Work out the finished part from the listing and answer in its coordinate system (mm). Face numbers are marked on the shaded views. Coordinates: 2 decimals unless noted, no trailing zeros. Order: outer loops, then holes, each group sorted by start corner. A loop starts at its lowest first (then second) coordinate and runs counter-clockwise, first axis right, second up. Notation, with made-up numbers: M 79,39.25 L 120,39.25 A28 cw 120,76.25 Z; hole C 75.5,75 d8. An arc over 180 degrees is marked long. Use a Markdown table: item, result.
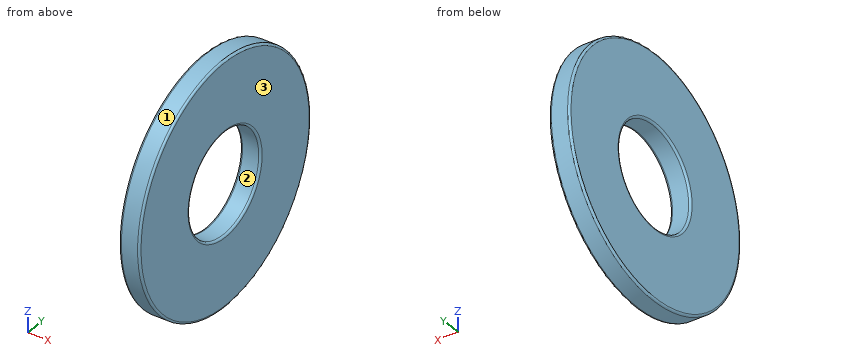
from build123d import *

# Parameters (mm, degrees)
F0_R     = 6
F0_R_2   = 2.5
F1_DEPTH = 1
F2_R     = 0.1
F3_R     = 0.1


with BuildPart() as f1:
    # F0 (on Right) → F1 (new body)
    with BuildSketch(Plane.YZ):
        Circle(F0_R)
        Circle(F0_R_2, mode=Mode.SUBTRACT)
    extrude(amount=F1_DEPTH)

    # F2
    f2_edges = [f1.edges().sort_by_distance(p)[0] for p in [
        (1, -6, 0),
        (0, -6, 0),
    ]]
    fillet(f2_edges, radius=F2_R)

    # F3
    f3_edges = [f1.edges().sort_by_distance(p)[0] for p in [
        (0, -2.5, 0),
        (1, -2.5, 0),
    ]]
    fillet(f3_edges, radius=F3_R)


solid = f1.part
(1) Straight lines are drawn through the part: L1, parallel to Z at x = 0.35, y = 0; L2, parallel to Y at x = 0.2, z = 1.25; L3, parallel to Y at x = 0.15, z = 1.5. For each, find the intervals that lie inside material, in ascending order.
Conclusion:
| item | result |
|---|---|
| L1 | -6 to -2.5, 2.5 to 6 |
| L2 | -5.87 to -2.17, 2.17 to 5.87 |
| L3 | -5.81 to -2, 2 to 5.81 |
(2) A cutting plane is placed at A-A (z = 0). Determine the outline of the cut face in (x, y).
Conclusion:
| item | result |
|---|---|
| outline | M 0,-5.9 A0.1 ccw 0.1,-6 L 0.9,-6 A0.1 ccw 1,-5.9 L 1,-2.6 A0.1 ccw 0.9,-2.5 L 0.1,-2.5 A0.1 ccw 0,-2.6 Z; M 0,2.6 A0.1 ccw 0.1,2.5 L 0.9,2.5 A0.1 ccw 1,2.6 L 1,5.9 A0.1 ccw 0.9,6 L 0.1,6 A0.1 ccw 0,5.9 Z |
(3) Determine the mould class of the marked faces 1, 2 and 3 for opening direction Y: pulls with the +Y half, pulls with the -Y half, needs draft (parallel to the pull), parting line crosses it, or undercut.
Conclusion:
| item | result |
|---|---|
| face 1 | parting line crosses it |
| face 2 | undercut |
| face 3 | needs draft |
(4) A cutting plane is placed at C-C (x = 0.7). Determine the outline of the cut face in (y, z), then the cut area to 3 significant figures.
Conclusion:
| item | result |
|---|---|
| outline | C 0,0 d12; hole C 0,0 d5 |
| area | 93.5 mm2 |
